Design review of the part built by this model. Coordinates are the model's own, in mm. Face numbers are marked on the shaded views. A direction names the side the tool comes from. Give positions to 0.01 mm unless a question says otherwise; leave off trailing zeros. Write each loop counter-clockwise with the first axis right and the second up, starting at its lowest first coordinate (ties: lowest second). Pieces come first, ordered by that corner, then holes. Notation, with made-up numbers: (26, 85.5) -> (37, 85.5) arc R35 cw to (37, 117.5) -> close; hole circle Ø1 at (27.25, 66.5). An arc over 180 degrees is marked (long way). Answer as a JSON object with one key per item and string values.
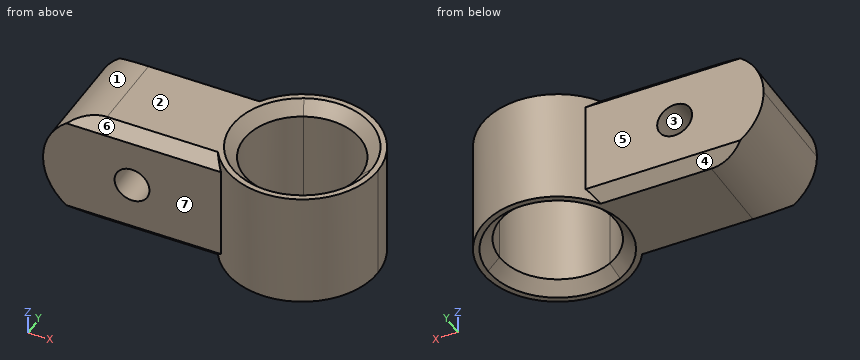
```python
from build123d import *

# Parameters (mm, degrees)
F1_DEPTH = 10
F3_D     = 3
F3_DEPTH = 30
F3_TIP   = 0.9012909285
F4_SIZE  = 1
F5_R     = 4.99999


# Not quite as in the source:
# - a fillet or chamfer is up to 0.001 mm smaller than in the source, because OpenCascade refuses the exact size


with BuildPart() as f1:
    # F0 (on Top) → F1 (new body)
    with BuildSketch(Plane.XY):
        with BuildLine():
            Line((5.3095842402, 4.5), (-10, 4.5))
            Line((-10, 4.5), (-10, -4.5))
            Line((-10, -4.5), (5.3095842402, -4.5))
            ThreePointArc((5.3095842402, -4.5), (3.5, 0), (5.3095842402, 4.5))
        make_face()
        with BuildLine():
            Line((7.8205505282, 4.5), (5.3095842402, 4.5))
            ThreePointArc((5.3095842402, 4.5), (3.5, 0), (5.3095842402, -4.5))
            Line((5.3095842402, -4.5), (7.8205505282, -4.5))
            ThreePointArc((7.8205505282, -4.5), (5, 0), (7.8205505282, 4.5))
        make_face()
        with BuildLine():
            ThreePointArc((16.5, 0), (12.4251079936, 6.0306592691), (5.3095842402, 4.5))
            Line((5.3095842402, 4.5), (7.8205505282, 4.5))
            ThreePointArc((7.8205505282, 4.5), (12.655442773, 4.2365816031), (15, 0))
            ThreePointArc((15, 0), (12.655442773, -4.2365816031), (7.8205505282, -4.5))
            Line((7.8205505282, -4.5), (5.3095842402, -4.5))
            ThreePointArc((5.3095842402, -4.5), (12.4251079936, -6.0306592691), (16.5, 0))
        make_face()
    extrude(amount=F1_DEPTH)

    # F3
    with Locations(Plane.XZ.offset(4.5)):
        with Locations((-2.3452078799, 5)):
            Hole(F3_D / 2, depth=F3_DEPTH)
            with Locations((0, 0, -(F3_DEPTH + F3_TIP / 2))):  # 118° drill point
                Cone(0, F3_D / 2, F3_TIP, mode=Mode.SUBTRACT)

    # F4
    f4_edges = [f1.edges().sort_by_distance(p)[0] for p in [
        (12.179449, -4.5, 10),
        (12.179449, -4.5, 0),
        (-2.345208, 4.5, 10),
        (-2.345208, -4.5, 10),
        (-2.345208, -4.5, 0),
        (-2.345208, 4.5, 0),
    ]]
    chamfer(f4_edges, length=F4_SIZE)

    # F5 (radius 5 in the source; OpenCascade refuses exactly that, so slightly less here)
    f5_edges = [f1.edges().sort_by_distance(p)[0] for p in [
        (-10, 0, 10),
        (-10, 0, 0),
    ]]
    fillet(f5_edges, radius=F5_R)


solid = f1.part
```
(1) We need section C-C, the plane y = 3.75. Give the number of separate pieces and of enclosed holes in the cut face, then the cut area to 3 significant figures.
Here are the results:
{"separate pieces": "2", "enclosed holes": "1", "area": "161 mm²"}
(2) Clearance check with flat-ended pins moving along their axes: pin 1 (2.5 mm diameter, centred on x = -0.5, z = 3.5, fed in from -Y); pin 2 (3 mm diameter, centred on x = -7, y = -3.5, fed in from -Z); pin 3 (1 mm diameter, centred on y = 0.5, z = 2, fed in from -X). State where each tip first meets the part, or that it passes through.
Here are the results:
{"pin 1": "stops at y = -4.5", "pin 2": "stops at z = 0.03", "pin 3": "stops at x = -9.33"}
(3) We need section B-B, the plane x = -2. State the section outline as (y, z) points, then the cut area to 3 significant figures.
Here are the results:
{"outline": "(-4.5, 1) -> (-3.5, 0) -> (3.5, 0) -> (4.5, 1) -> (4.5, 3.54) -> (-4.5, 3.54) -> close; (-4.5, 6.46) -> (4.5, 6.46) -> (4.5, 9) -> (3.5, 10) -> (-3.5, 10) -> (-4.5, 9) -> close", "area": "61.7 mm²"}
(4) For the marked faces 4, 5, 6 and 7, list the 3-axis set-ups (+Z, -Z, +X, -X, +Y, -Y) from which the entire face can be reached by the end or side of a thin tool; tool diameter is ignored.
Here are the results:
{"face 4": "-Z, -X, +Y", "face 5": "+Z, -Z, -X, +Y", "face 6": "+Z, -X, -Y", "face 7": "+Z, -Z, -X, -Y"}
(5) We need section A-A, the plane z = 4.25. State the section outline as (x, y) points, then the cut area to 3 significant figures.
Here are the results:
{"outline": "(-9.94, -4.5) -> (-3.64, -4.5) -> (-3.64, 4.5) -> (-9.94, 4.5) -> close; (-1.05, -4.5) -> (5.31, -4.5) arc R6.5 ccw (long way) to (5.31, 4.5) -> (-1.05, 4.5) -> close; hole circle Ø10 at (10, 0)", "area": "157 mm²"}
(6) For line 1 along Y through (x, z) = (9.75, 6); line 2 along X through (y, z) = (-1.75, 3.75); line 3 along Y through (x, z) = (-7, 7.25), list the stretches that pass through material, from the lowest coordinate up.
Here are the results:
{"line 1": "y = -6.5 to -4.99, 4.99 to 6.5", "line 2": "x = -9.84 to -3.17, -1.52 to 5.32, 14.68 to 16.26", "line 3": "y = -4.5 to 4.5"}
(7) The part is to be moulded in two halves that separate along X. For the marked faces 1, 2 and 3, say which applies: +X half, -X half, draft (parallel to the pull), parting line (faces both ways), or undercut.
Here are the results:
{"face 1": "-X half", "face 2": "draft", "face 3": "undercut"}
(8) We need section D-D, the plane z = 6.75. State the section outline as (x, y) points, then the cut area to 3 significant figures.
Here are the results:
{"outline": "(-9.68, -4.5) -> (5.31, -4.5) arc R6.5 ccw (long way) to (5.31, 4.5) -> (-9.68, 4.5) -> close; hole circle Ø10 at (10, 0)", "area": "178 mm²"}
